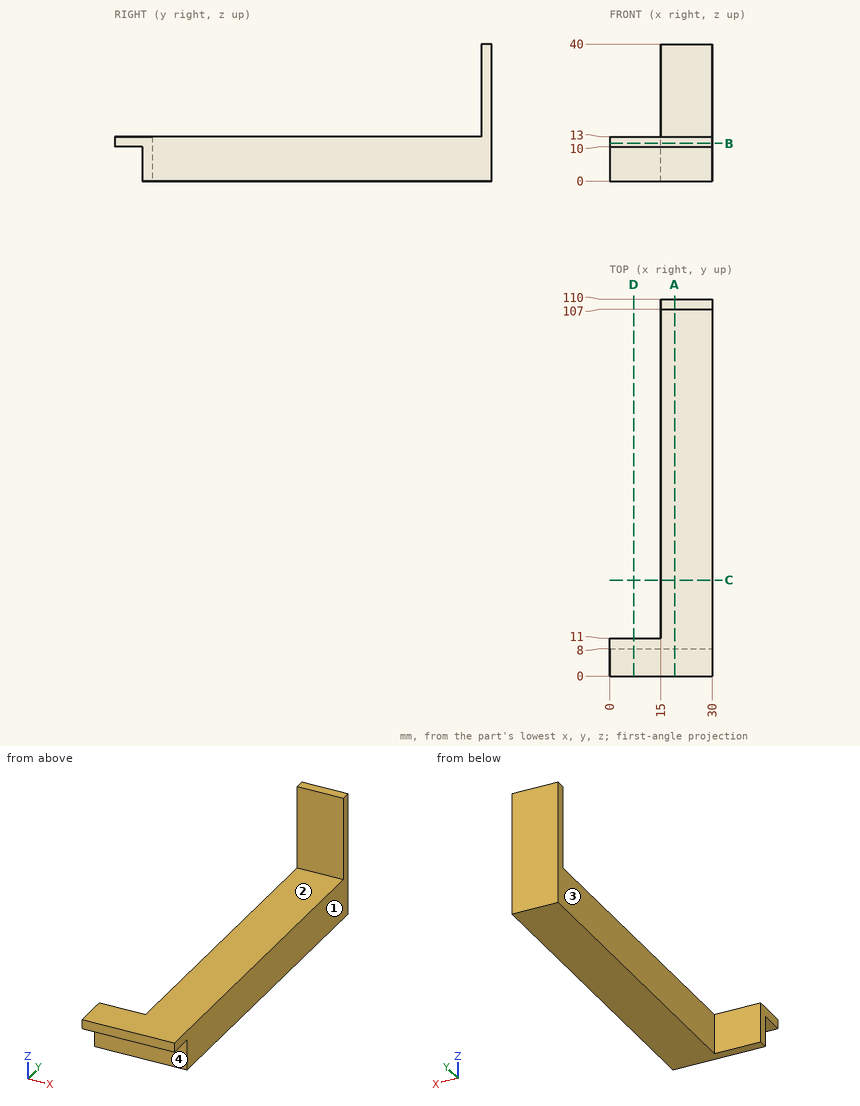
Study the drawing (mm; zero at the part's minimum x, y, z) and answer. A direction names the side the tool comes from. Coordinates: 2 decimals unless noted, no trailing zeros. Order: outer loops, then holes, each group sorted by start corner. A loop starts at its lowest first (then second) coordinate and runs counter-clockwise, first axis right, second up. Notation, with made-up numbers: (82.5, 10.25) -> (89.5, 10.25) arc R8 cw to (89.5, 14.25) -> close; hole circle Ø2 at (13.25, -23). An arc over 180 degrees is marked (long way). Answer in a Markdown table with one row per item. Add a question column.
Item 1: Find the intervals of material crossed by L1, parallel to Y at x = 22.25, z = 22; L2, parallel to Y at x = 7.75, z = 4; L3, parallel to Z at x = 21, y = 105.5, in increasing order. Write a range as from..to.
Item 2: Find section A-A (x = 19). Write down the section's boundary in (y, z).
Item 3: Find section D-D (x = 7). Write down the section's boundary in (y, z), then the cut area to 3 significant figures.
Item 4: Each of these flat-tipped pins is pushed along its axis until it touches: P1, Ø10, axis at x = 20.5, y = 47, coming from the +Z side; P2, Ø9, axis at x = 7.5, y = 4.5, coming from the -Z side; P3, Ø14.5, axis at x = 6, z = 9.5, coming from the +Y side; P4, Ø8, axis at x = 13, z = 3, coming from the -Y side. Where does it stop, or does it pass through?
Item 5: Find section B-B (z = 11). Write down the section's boundary in (x, y).
Item 6: Find section C-C (y = 28). Write down the section's boundary in (x, z).
Item 7: Which of the six approach directions +Z, -Z, +X, -X, +Y, -Y give full straight-line access (tool end or side, diameter ignored) to the marked faces 1, 2, 3 and 4?
Result set:
| question | item | result |
|---|---|---|
| 1 | L1 | y = 107..110 |
| 1 | L2 | y = 8..11 |
| 1 | L3 | z = 0..13 |
| 2 | outline | (0, 10) -> (8, 10) -> (8, 0) -> (110, 0) -> (110, 40) -> (107, 40) -> (107, 13) -> (0, 13) -> close |
| 3 | outline | (0, 10) -> (8, 10) -> (8, 0) -> (11, 0) -> (11, 13) -> (0, 13) -> close |
| 3 | area | 63.0 mm² |
| 4 | P1 | stops at z = 13 |
| 4 | P2 | stops at z = 0 |
| 4 | P3 | stops at y = 11 |
| 4 | P4 | stops at y = 8 |
| 5 | outline | (0, 0) -> (30, 0) -> (30, 110) -> (15, 110) -> (15, 11) -> (0, 11) -> close |
| 6 | outline | (15, 0) -> (30, 0) -> (30, 13) -> (15, 13) -> close |
| 7 | face 1 | +Z, -Z, +X, +Y, -Y |
| 7 | face 2 | +Z, +X, -X, -Y |
| 7 | face 3 | +Z, -Z, -X, +Y |
| 7 | face 4 | -Z, +X, -X, -Y |
